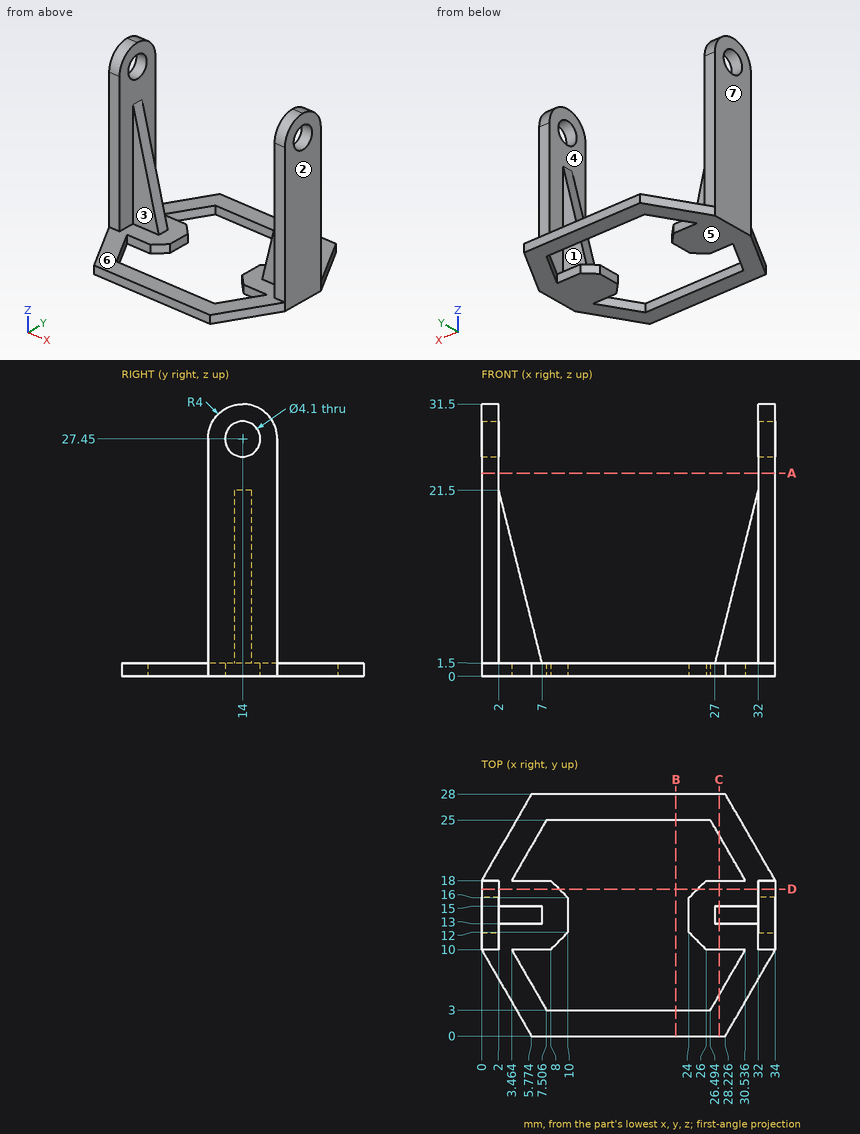
The figure shows three views and two pictorial views of one solid part (mm, origin at its lowest corner). Answer the questions. A direction names the side the tool comes from. Coordinates: 2 decimals unless noted, no trailing zeros. Loops run counter-clockwise (first coordinate to the right, second up) from the corner with the lowest first, then second, coordinate; pieces in that order, holes last. Notation, with made-up numbers: M 66.25,80.25 L 119.25,80.25 A19 cw 119.25,96.25 Z; hole C -3.5,75 d9. An arc over 180 degrees is marked long. Answer as CSV lines item,"result". Start each with the question number.
(1) The part is cut by section D-D (y = 17). Give the vertices of the cut face in (x, z) (1 decimal).
(2) The part is cut by section B-B (x = 22.5). Give the vertices of the cut face in (y, z).
(3) The part is cut by section C-C (x = 27.5). Give the vertices of the cut face in (y, z).
(4) Find the intervals of material crossed by L1, parallel to Z at x = 1.3, y = 14; L2, parallel to X at y = 15.5, z = 24; L3, parallel to Y at x = 1, z = 27, in increasing order. Write a range as [from, to].
(5) Given pin 1 (1.6 mm diameter, centred on x = 33, z = 10, fed in from +Y); pin 2 (6 mm diameter, centred on x = 17.5, y = 23, fed in from +Z); pin 3 (3.5 mm diameter, centred on y = 14, z = 27.45, fed in from +X); pin 4 (0.6 mm diameter, centred on x = 1, z = 9.5, fed in from -Y), each flat-ended and moving along its own axis, determine where each tip first touches the part or whether it passes through.
(6) For the marked faces 1, 2, 3 and 4, determine the directions among +Z, -Z, +X, -X, +Y, -Y from which every point of the face is accessible in a straight line to the end or side of a thin tool.
(7) The part is cut by section A-A (z = 23.5). Give the vertices of the cut face in (x, y), and give its area (3 significant figures).
(8) The mould has two halves that part along X. Classify the marked faces 5, 6 and 7: pulls with the +X half, pulls with the -X half, needs draft (parallel to the pull), parting line crosses it, or undercut.
Determined:
1,outline,"M 0,0 L 9,0 L 9,1.5 L 2,1.5 L 2,30.1 L 0,30.1 Z; M 25,0 L 34,0 L 34,30.1 L 32,30.1 L 32,1.5 L 25,1.5 Z"
2,outline,"M 0,0 L 3,0 L 3,1.5 L 0,1.5 Z; M 25,0 L 28,0 L 28,1.5 L 25,1.5 Z"
3,outline,"M 0,0 L 4.74,0 L 4.74,1.5 L 0,1.5 Z; M 10,0 L 18,0 L 18,1.5 L 15,1.5 L 15,3.5 L 13,3.5 L 13,1.5 L 10,1.5 Z; M 23.26,0 L 28,0 L 28,1.5 L 23.26,1.5 Z"
4,L1,"[0, 25.4], [29.5, 31.5]"
4,L2,"[0, 2], [32, 34]"
4,L3,"[10, 12], [16, 18]"
5,pin 1,"y = 18"
5,pin 2,"z = 1.5"
5,pin 3,"through"
5,pin 4,"y = 10"
6,face 1,"+Z, +Y"
6,face 2,"+Z, -Z, +X, +Y, -Y"
6,face 3,"+Z, -Y"
6,face 4,"+Z"
7,outline,"M 0,10 L 2,10 L 2,18 L 0,18 Z; M 32,10 L 34,10 L 34,18 L 32,18 Z"
7,area,"32.0 mm2"
8,face 5,"needs draft"
8,face 6,"undercut"
8,face 7,"pulls with the -X half"
